Autodesk Inventor part; units mm, degrees
ref_plane "YZ Plane" through (0, 0, 0) normal (1, 0, 0) x (0, 1, 0)
ref_plane "XZ Plane" through (0, 0, 0) normal (0, 1, 0) x (-1, 0, 0)
ref_plane "XY Plane" through (0, 0, 0) normal (0, 0, 1) x (1, 0, 0)
sketch "Sketch1" plane through (0, 0, 0) normal (0, 0, 1) x (1, 0, 0)
  circle A0 centre (0, 0) radius 20.75
  dimension "d0" = 41.5
extrude "Extrusion1" add sketch "Sketch1" along normal blind 26.7
sketch "Sketch2" plane through (0, 0, 26.7) normal (0, 0, 1) x (1, 0, 0)
  circle A0 centre (-15.1554, 8.75) radius 2
  circle A1 centre (15.1554, 8.75) radius 2
  circle A2 centre (0, -17.5) radius 2
  circle A3 centre (0, 0) radius 17.5 construction
  line L0 (0, 0) -> (-15.1554, 8.75) construction
  line L1 (0, 0) -> (15.1554, 8.75) construction
  line L2 (0, 0) -> (0, -17.5) construction
  dimension "d3" = 35
  dimension "d4" = 120
  dimension "d5" = 120
  dimension "d6" = 4
extrude "Extrusion2" cut sketch "Sketch2" against normal blind 20
properties part number "Hoverboard Frame"
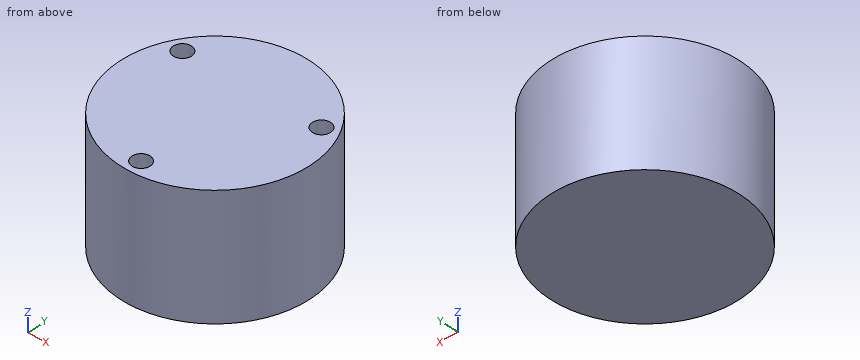
The listing builds one solid part. Answer for the finished solid, in the listing's coordinates (mm). Coordinates: 2 decimals unless noted, no trailing zeros. Order: outer loops, then holes, each group sorted by start corner. A loop starts at its lowest first (then second) coordinate and runs counter-clockwise, first axis right, second up.
Q1. A cutting plane is placed at C-C, the plane y = 8.75. Write down the section's boundary in (x, z), and give its area (3 significant figures).
Q2. A cutting plane is placed at D-D, the plane z = 2.25. Write down the section's boundary in (x, y), and give its area (3 significant figures).
Q3. Given P1, Ø3, axis at x = -12.5, z = 20.5, coming from the +Y side; P2, Ø8, axis at x = 3, z = 6, coming from the +Y side; P3, Ø2, axis at x = -15, y = 8, coming from the +Z side, each flat-ended and moving along its own axis, determine where each tip first touches the part or whether it passes through.
Q4. Consider line 1 (Y direction, x = 0, z = 20.5); line 2 (X direction, y = 9.5, z = 19.25); line 3 (Y direction, x = -16, z = 8). Determine where each line is inside the solid, lowest interval first.
Q5. A cutting plane is placed at A-A, the plane x = 0. Write down the section's boundary in (y, z), and give its area (3 significant figures).
Q6. A cutting plane is placed at B-B, the plane z = 21.75. Write down the section's boundary in (x, y).
Answers follow:
1. outline: (-18.81, 0) - (18.81, 0) - (18.81, 26.7) - (17.16, 26.7) - (17.16, 6.7) - (13.16, 6.7) - (13.16, 26.7) - (-13.16, 26.7) - (-13.16, 6.7) - (-17.16, 6.7) - (-17.16, 26.7) - (-18.81, 26.7) - close
1. area: 845 mm2
2. outline: circle Ø41.5 at (0, 0)
2. area: 1,350 mm2
3. P1: stops at y = 17.59
3. P2: stops at y = 20.75
3. P3: stops at z = 6.7
4. line 1: y = -20.75 to -19.5, -15.5 to 20.75
4. line 2: x = -18.45 to -17.01, -13.3 to 13.3, 17.01 to 18.45
4. line 3: y = -13.21 to 6.94, 10.56 to 13.21
5. outline: (-20.75, 0) - (20.75, 0) - (20.75, 26.7) - (-15.5, 26.7) - (-15.5, 6.7) - (-19.5, 6.7) - (-19.5, 26.7) - (-20.75, 26.7) - close
5. area: 1,030 mm2
6. outline: circle Ø41.5 at (0, 0); hole circle Ø4 at (-15.16, 8.75); hole circle Ø4 at (0, -17.5); hole circle Ø4 at (15.16, 8.75)
